```python
from build123d import *

# Parameters (mm, degrees)
SKETCH_W     = 32
SKETCH_H     = 200
PAD_DEPTH    = 50
SKETCH001_W  = 26
SKETCH001_H  = 200
POCKET_DEPTH = 10
FILLET_R     = 1
FILLET001_R  = 1
FILLET002_R  = 1
FILLET003_R  = 1


with BuildPart() as part:
    # Sketch → Pad (new body)
    with BuildSketch(Plane.XY):
        with Locations((16, 0)):
            Rectangle(SKETCH_W, SKETCH_H)
    extrude(amount=PAD_DEPTH)

    # Sketch001 (on Face6 of Pad) → Pocket (cut)
    with BuildSketch(Plane.XY.offset(50)):
        with Locations((16, -3)):
            Rectangle(SKETCH001_W, SKETCH001_H)
    extrude(amount=-POCKET_DEPTH, mode=Mode.SUBTRACT)

    # Fillet
    fillet_edges = [part.edges().sort_by_distance(p)[0] for p in [
        (32, -100, 25),
    ]]
    fillet(fillet_edges, radius=FILLET_R)

    # Fillet001
    fillet001_edges = [part.edges().sort_by_distance(p)[0] for p in [
        (0, -100, 25),
    ]]
    fillet(fillet001_edges, radius=FILLET001_R)

    # Fillet002
    fillet002_edges = [part.edges().sort_by_distance(p)[0] for p in [
        (0, 100, 25),
    ]]
    fillet(fillet002_edges, radius=FILLET002_R)

    # Fillet003
    fillet003_edges = [part.edges().sort_by_distance(p)[0] for p in [
        (32, 100, 25),
    ]]
    fillet(fillet003_edges, radius=FILLET003_R)


solid = part.part
```
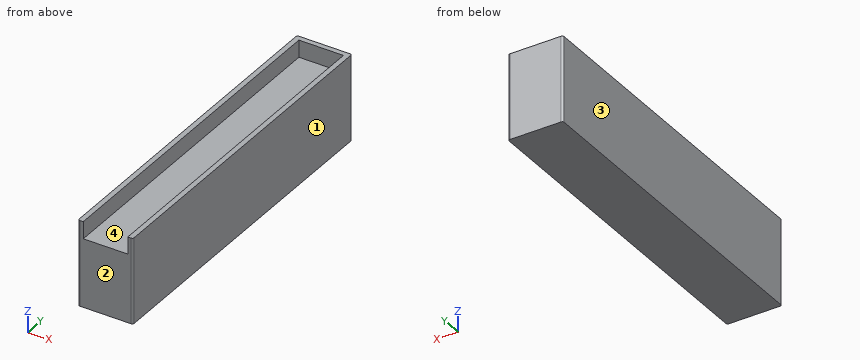
Work out the finished part from the listing and answer in its coordinate system (mm). Face numbers are marked on the shaded views. Coordinates: 2 decimals unless noted, no trailing zeros. Write each loop counter-clockwise with the first axis right and the second up, starting at its lowest first coordinate (ties: lowest second). Pieces come first, ordered by that corner, then holes.
Q1. A cutting plane is placed at A-A, the plane x = 12.5. Give the vertices of the cut face in (y, z), then the cut area to 3 significant figures.
Q2. Find the intervals of material crossed by line 1 (X direction, y = 12, z = 40.5); line 2 (Z direction, x = 14, y = 37.5), in increasing order.
Q3. A cutting plane is placed at B-B, the plane z = 43. Give the vertices of the cut face in (x, y), then the cut area to 3 significant figures.
Q4. Each of these flat-tipped pins is pushed along its axis until it touches: pin 1 Ø1 at (x, y) = (19.5, -25.5) entering from -Z; pin 2 Ø3 at (x, z) = (11, 43.5) entering from -Y. Where does it stop, or does it pass through?
Q5. A cutting plane is placed at C-C, the plane y = 31. Give the vertices of the cut face in (x, z), then the cut area to 3 significant figures.
Q6. Determine the mould class of the marked faces 1, 2, 3 and 4 for opening direction X: released by +X, released by -X, zero draft, split by the parting line, or undercut.
Findings below:
1. outline: (-100, 0) - (100, 0) - (100, 50) - (97, 50) - (97, 40) - (-100, 40) - close
1. area: 8,030 mm2
2. line 1: x = 0 to 3, 29 to 32
2. line 2: z = 0 to 40
3. outline: (0, -99) arc R1 ccw to (1, -100) - (3, -100) - (3, 97) - (29, 97) - (29, -100) - (31, -100) arc R1 ccw to (32, -99) - (32, 99) arc R1 ccw to (31, 100) - (1, 100) arc R1 ccw to (0, 99) - close
3. area: 1,280 mm2
4. pin 1: stops at z = 0
4. pin 2: stops at y = 97
5. outline: (0, 0) - (32, 0) - (32, 50) - (29, 50) - (29, 40) - (3, 40) - (3, 50) - (0, 50) - close
5. area: 1,340 mm2
6. face 1: released by +X
6. face 2: zero draft
6. face 3: released by -X
6. face 4: undercut
